Could you check a few things on this model? Use its own coordinates, in mm. Face numbers are marked on the shaded views. A direction names the side the tool comes from. Give positions to 0.01 mm unless a question says otherwise; leave off trailing zeros. Loops run counter-clockwise (first coordinate to the right, second up) from the corner with the lowest first, then second, coordinate; pieces in that order, holes last. Notation, with made-up numbers: (58, 0) -> (63, 0) arc R17 ccw to (63, 17) -> close; hole circle Ø2 at (39.25, 21). An arc over 180 degrees is marked (long way). Write each question's results on one line, items separated by ' | '. Start each with the question number.
Q1. Will these pins go through, and if not, where does the flat tip stop? P1, Ø5, axis at y = 0.5, z = 14.5, coming from the -X side (3 decimals); P2, Ø2, axis at x = -2.5, z = 24.5, coming from the +Y side; P3, Ø0.8, axis at y = 2.5, z = 0.5, coming from the +X side; P4, Ø2.5, axis at x = 0, y = 0, coming from the -Z side.
Q2. If we section it at D-D, the plane x = 3.75: List the corners of the cut face in (y, z) for me.
Q3. Which directions (+Z, -Z, +X, -X, +Y, -Y) give clear straight access to the entire face, cutting with the end or side of a thin tool? Please do the marked faces 1 and 2.
Q4. If we section it at C-C, the plane y = -3.5: List the corners of the cut face in (x, z) for me, plus the area to 3 significant figures.
Q5. If I drill on line 1 along Y through (x, z) = (0, 9) (1 decimal); line 2 along Y through (x, z) = (0, 30.1) (3 decimals); line 3 along Z through (x, y) = (-0.5, 3.75), over which ranges is the centre line in solid material (lowest first)?
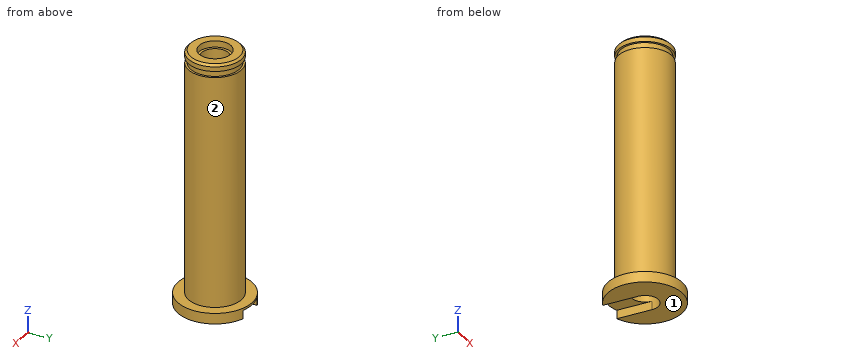
from build123d import *

# Parameters (mm, degrees)
SKETCH2_R           = 4.445
BOSS_EXTRUDE1_DEPTH = 1.27
SKETCH3_R           = 3.175
BOSS_EXTRUDE2_DEPTH = 29.21
SKETCH4_R           = 1.5875
CUT_EXTRUDE1_DEPTH  = 37.592
SKETCH5_R           = 1.905
CUT_EXTRUDE2_DEPTH  = 0.762
SKETCH6_W           = 3.175
SKETCH6_H           = 5.873367688
CUT_EXTRUDE3_DEPTH  = 1.016
CUT_EXTRUDE5_START  = -0.7366
SKETCH7_R           = 3.175
SKETCH7_R_2         = 2.921
CUT_EXTRUDE5_DEPTH  = 0.7366
CHAMFER1_SIZE       = 0.254


with BuildPart() as part:
    # Sketch2 → Boss-Extrude1 (new body)
    with BuildSketch(Plane.XY):
        Circle(SKETCH2_R)
    extrude(amount=BOSS_EXTRUDE1_DEPTH)

    # Sketch3 → Boss-Extrude2 (add)
    with BuildSketch(Plane.XY.offset(1.27)):
        with Locations(Location((0, 0, 0), (0, 0, 180))):
            Circle(SKETCH3_R)
    extrude(amount=BOSS_EXTRUDE2_DEPTH)

    # Sketch4 → Cut-Extrude1 (cut)
    with BuildSketch(Plane.XY.offset(30.48)):
        Circle(SKETCH4_R)
    extrude(amount=-CUT_EXTRUDE1_DEPTH, mode=Mode.SUBTRACT)

    # Sketch5 → Cut-Extrude2 (cut)
    with BuildSketch(Plane.XY.offset(30.48)):
        Circle(SKETCH5_R)
    extrude(amount=-CUT_EXTRUDE2_DEPTH, mode=Mode.SUBTRACT)

    # Sketch6 → Cut-Extrude3 (cut)
    with BuildSketch(Plane(origin=(0, 0, 0), x_dir=(-1, 0, 0), z_dir=(0, 0, -1))):
        with Locations((0, 2.936683844)):
            Rectangle(SKETCH6_W, SKETCH6_H)
    extrude(amount=-CUT_EXTRUDE3_DEPTH, mode=Mode.SUBTRACT)

    # Sketch7 → Cut-Extrude5 (cut)
    with BuildSketch(Plane.XY.offset(29.6799).offset(CUT_EXTRUDE5_START)):
        with Locations(Location((0, 0, 0), (0, 0, 180))):
            Circle(SKETCH7_R)
        Circle(SKETCH7_R_2, mode=Mode.SUBTRACT)
    extrude(amount=CUT_EXTRUDE5_DEPTH, mode=Mode.SUBTRACT)

    # Chamfer1
    chamfer1_edges = [part.edges().sort_by_distance(p)[0] for p in [
        (3.175, 0, 30.48),
    ]]
    chamfer(chamfer1_edges, length=CHAMFER1_SIZE)


solid = part.part
Final values:
1) P1: stops at x = -3.175 | P2: stops at y = 2.8 | P3: stops at x = 3.92 | P4: passes through
2) outline: (-2.39, 0) -> (2.39, 0) -> (2.39, 1.27) -> (-2.39, 1.27) -> close
3) face 1: -Z, +X, -X, +Y, -Y | face 2: +Z
4) outline: (-2.74, 0) -> (2.74, 0) -> (2.74, 1.27) -> (-2.74, 1.27) -> close | area: 6.96 mm²
5) line 1: y = -3.2 to -1.6, 1.6 to 3.2 | line 2: y = -3.175 to -1.905, 1.905 to 3.175 | line 3: z = 1.02 to 1.27
